Geometry check sheet. Reference: drawing and pictorial views, mm from the part's lowest x, y, z. A direction names the side the tool comes from. Round coordinates to 2 decimals unless told otherwise and drop trailing zeros. Order: outer loops, then holes, each group sorted by start corner. A loop starts at its lowest first (then second) coordinate and runs counter-clockwise, first axis right, second up.
Q1. Cross-section at C-C on z = 19. Record the cut outline in (x, y).
Q2. Scan lines: probe 1 along Z at (x, y) = (1.6, 6); probe 2 along Y at (x, z) = (4.8, 35.5); probe 3 along Z at (x, y) = (0.2, 46.5). Record each from-to range of solid material in increasing order.
Q3. Cross-section at B-B on x = 0.8. Record the cut outline in (y, z) (3 decimals), then the cut area to 3 significant figures.
Q4. Depth check by flat-ended pin: P1, Ø1.5, axis at x = 1.5, z = 20.5, coming from the -Y side; P2, Ø2.5, axis at y = 3.175, z = 34.925, coming from the +X side; P3, Ø1.5, axis at x = 2, z = 19, coming from the +Y side; P4, Ø6, axis at y = 41, z = 9, coming from the -X side. Enter the tip coordinate at first touch or a pass-through.
Q5. Set-up check for the marked faces 1, 2 and 3: record each of +Z, -Z, +X, -X, +Y, -Y from which the full face is reachable in a straight line by a thin tool's end or side.
Q6. Mould release check, pull along Z, two halves, no side actions. Record for the marked faces 4, 5, 6 and 7: +Z half, -Z half, draft (parallel to the pull), parting line (faces both ways), or undercut.
Q7. Cross-section at A-A on y = 47. Record the cut outline in (x, z).
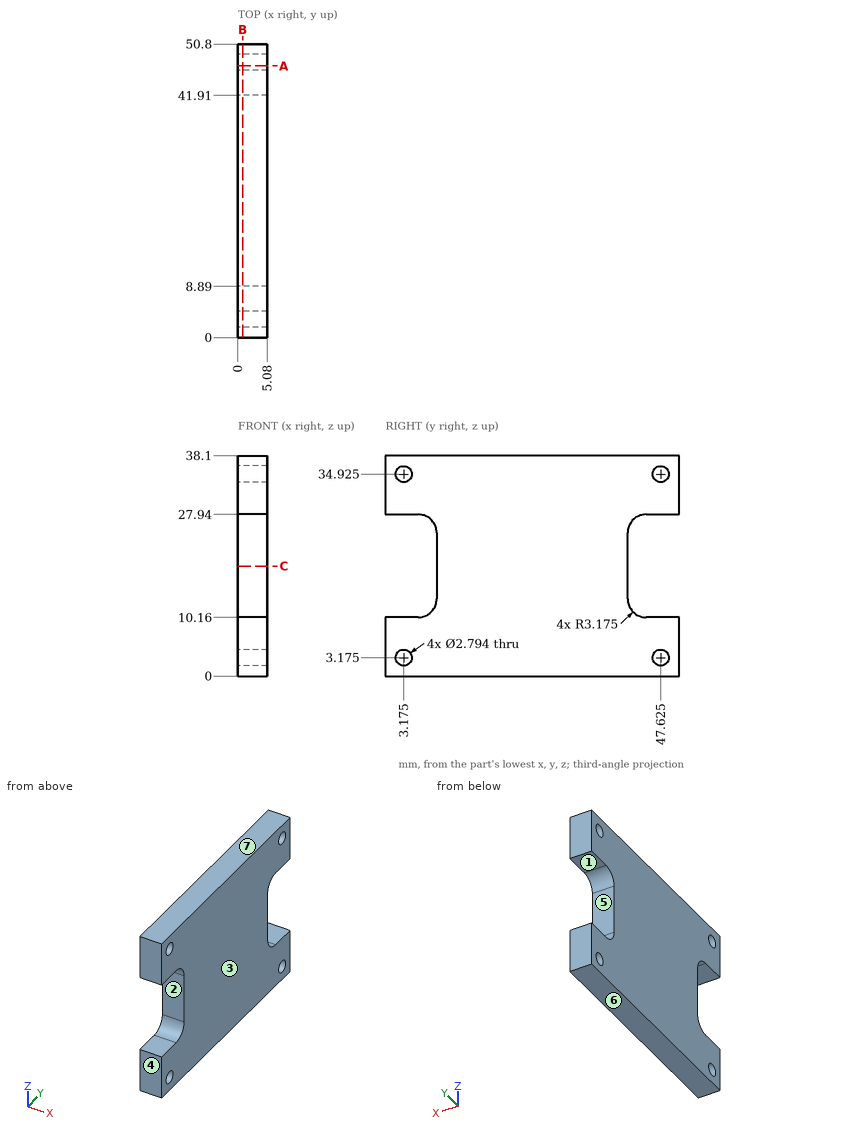
Results found:
1. outline: (0, 8.89) - (5.08, 8.89) - (5.08, 41.91) - (0, 41.91) - close
2. probe 1: z = 0 to 10.17, 27.93 to 38.1
2. probe 2: y = 0 to 1.9, 4.45 to 46.35, 48.9 to 50.8
2. probe 3: z = 0 to 2.35, 4 to 10.16, 27.94 to 34.1, 35.75 to 38.1
3. outline: (0, 0) - (50.8, 0) - (50.8, 10.16) - (45.085, 10.16) arc R3.175 cw to (41.91, 13.335) - (41.91, 24.765) arc R3.175 cw to (45.085, 27.94) - (50.8, 27.94) - (50.8, 38.1) - (0, 38.1) - (0, 27.94) - (5.715, 27.94) arc R3.175 cw to (8.89, 24.765) - (8.89, 13.335) arc R3.175 cw to (5.715, 10.16) - (0, 10.16) - close; hole circle Ø2.794 at (3.175, 3.175); hole circle Ø2.794 at (3.175, 34.925); hole circle Ø2.794 at (47.625, 3.175); hole circle Ø2.794 at (47.625, 34.925)
3. area: 1,600 mm2
4. P1: stops at y = 8.89
4. P2: passes through
4. P3: stops at y = 41.91
4. P4: stops at x = 0
5. face 1: +X, -X, +Y
5. face 2: +X, -X, -Y
5. face 3: +Z, -Z, +X, +Y, -Y
6. face 4: draft
6. face 5: undercut
6. face 6: -Z half
6. face 7: +Z half
7. outline: (0, 0) - (5.08, 0) - (5.08, 1.93) - (0, 1.93) - close; (0, 4.42) - (5.08, 4.42) - (5.08, 10.16) - (0, 10.16) - close; (0, 27.94) - (5.08, 27.94) - (5.08, 33.68) - (0, 33.68) - close; (0, 36.17) - (5.08, 36.17) - (5.08, 38.1) - (0, 38.1) - close
